Build history of the part. All positions in model axes, mm. Face numbers are marked on the shaded views. A direction names the side the tool comes from. Coordinates: 2 decimals unless noted, no trailing zeros. Loops run counter-clockwise (first coordinate to the right, second up) from the corner with the lowest first, then second, coordinate; pieces in that order, holes last.
Item 1: Flat gauge pins, fed straight in: pin 1 (19 mm diameter, centred on x = 1, y = 11.5, fed in from +Z); pin 2 (10 mm diameter, centred on y = 38.5, z = 6.5, fed in from +X); pin 3 (4 mm diameter, centred on x = -24, z = -1.5, fed in from +Y); pin 4 (10.5 mm diameter, centred on y = 19.5, z = 9.5, fed in from -X). Where does each tip first touch, or does it go through?
Item 2: Cut at A-A (x = 2). List the corners of the cut face in (y, z).
Item 3: 3-axis set-ups, long thin cutter, end or side, ignore diameter. For the marked faces 1, 2, 3, 4 and 5: which of +Z, -Z, +X, -X, +Y, -Y reach the whole face in a straight line?
Item 4: Mould opens along Y. For the marked faces 6, 7 and 8 say: released by +Y, released by -Y, zero draft, split by the parting line, or undercut.
Item 5: Cut at B-B (y = 20). List the corners of the cut face in (x, z).
Item 6: Drill centre lines: line 1 along X through (y, z) = (28, 4.25); line 2 along Z through (x, y) = (27, 4.5); line 3 along X through (y, z) = (5, 0.75). Where is each one in solid material? Low to high.
from build123d import *

# Parameters (mm, degrees)
SKETCH13_W              = 80
SKETCH13_H              = 8
BOSS_EXTRUDE9_DEPTH     = 6.5
SKETCH14_W              = 15
SKETCH14_H              = 3.4999999999999996
CUT_EXTRUDE1_DEPTH      = 41.72161588149469
SKETCH15_W              = 35
SKETCH15_H              = 8
BOSS_EXTRUDE10_DEPTH    = 15
BOSS_EXTRUDE11_DEPTH    = 35
SKETCH17_R              = 3.0000000000000036
SKETCH17_R_2            = 3
BOSS_EXTRUDE12_DEPTH    = 1
SKETCH20_R              = 1.3000000000000023
CUT_EXTRUDE2_DEPTH      = 68.35348577458582
CUT_EXTRUDE3_DEPTH      = 68.33334117794962
CUT_EXTRUDE3_DEPTH_BACK = 68.33334117794962
CUT_EXTRUDE4_DEPTH      = 68.3333411779496
FILLET2_R               = 1.5
CHAMFER1_SIZE           = 1
FILLET3_R               = 20
FILLET4_R               = 2.5


with BuildPart() as part:
    # Sketch13 → Boss-Extrude9 (new body)
    with BuildSketch(Plane(origin=(0, 0, 0), x_dir=(1, 0, 0), z_dir=(0, 1, 0))):
        Rectangle(SKETCH13_W, SKETCH13_H)
    extrude(amount=BOSS_EXTRUDE9_DEPTH)

    # Sketch14 → Cut-Extrude1 (cut, through all)
    with BuildSketch(Plane(origin=(0, 6.5, 0), x_dir=(1, 0, 0), z_dir=(0, 1, 0))):
        Polygon((-35, -1.75), (-20, -1.7499999999999998), (-20, 1.7499999999999998), (-35, 1.75), align=None)
        with Locations((27.5, 0)):
            Rectangle(SKETCH14_W, SKETCH14_H)
    extrude(amount=-CUT_EXTRUDE1_DEPTH, mode=Mode.SUBTRACT)

    # Sketch15 → Boss-Extrude10 (add)
    with BuildSketch(Plane(origin=(0, 6.5, 0), x_dir=(1, 0, 0), z_dir=(0, 1, 0))):
        Rectangle(SKETCH15_W, SKETCH15_H)
    extrude(amount=BOSS_EXTRUDE10_DEPTH)

    # Sketch16 → Boss-Extrude11 (add)
    with BuildSketch(Plane.ZY.offset(17.5)):
        Polygon((4, 21.5), (16.678547852220913, 48.689233611099525), (10.107397413474738, 51.75341138357542), (-4, 21.5), align=None)
    extrude(amount=-BOSS_EXTRUDE11_DEPTH)

    # Sketch17 → Boss-Extrude12 (add)
    with BuildSketch(Plane(origin=(0, 2.307944309631712, -4.949402544155895), x_dir=(1, 0, 0), z_dir=(0, -0.42261826174069717, 0.9063077870366509))):
        with Locations(Location((-10.500000000000005, 47.17609046825079, 0), (0, 0, 90))):
            Circle(SKETCH17_R)
        with Locations(Location((10.499999999999995, 47.17609046825079, 0), (0, 0, 90))):
            Circle(SKETCH17_R_2)
        with Locations(Location((10.499999999999995, 34.67609046825079, 0), (0, 0, 90))):
            Circle(SKETCH17_R_2)
        with Locations(Location((-10.500000000000005, 34.67609046825079, 0), (0, 0, 90))):
            Circle(SKETCH17_R)
    extrude(amount=BOSS_EXTRUDE12_DEPTH)

    # Sketch20 → Cut-Extrude2 (cut, through all)
    with BuildSketch(Plane(origin=(0, 1.885326047891013, -4.043094757119239), x_dir=(1, 0, 0), z_dir=(0, -0.4226182617406972, 0.906307787036651))):
        with Locations(Location((-10.500000000000005, 47.176090468250806, 0), (0, 0, 270))):
            Circle(SKETCH20_R)
        with Locations(Location((10.499999999999995, 47.176090468250806, 0), (0, 0, 270))):
            Circle(SKETCH20_R)
        with Locations(Location((10.499999999999995, 34.67609046825079, 0), (0, 0, 270))):
            Circle(SKETCH20_R)
        with Locations(Location((-10.500000000000005, 34.67609046825079, 0), (0, 0, 270))):
            Circle(SKETCH20_R)
    extrude(amount=-CUT_EXTRUDE2_DEPTH, mode=Mode.SUBTRACT)

    # Sketch21 → Cut-Extrude3 (cut, two sides: drawn at the far end of the back side and taken through both)
    with BuildSketch(Plane(origin=(0, 2.307944309631711, -4.949402544155892), x_dir=(1, 0, 0), z_dir=(0, -0.4226182617406972, 0.906307787036651)).offset(-CUT_EXTRUDE3_DEPTH_BACK)):
        Polygon((-11.500000000000002, 9.676090468250791), (11.499999999999998, 9.676090468250791), (11.499999999999995, 29.67609046825079), (-11.500000000000002, 29.67609046825079), align=None)
    extrude(amount=CUT_EXTRUDE3_DEPTH + CUT_EXTRUDE3_DEPTH_BACK, mode=Mode.SUBTRACT)

    # Sketch22 → Cut-Extrude4 (cut, through all)
    with BuildSketch(Plane(origin=(0, 2.307944309631712, -4.949402544155895), x_dir=(1, 0, 0), z_dir=(0, -0.42261826174069717, 0.9063077870366509))):
        Polygon((-6.000000000000002, 47.676090468250806), (6.000000000000002, 47.676090468250806), (6, 29.676090468250802), (-6, 29.676090468250802), align=None)
    extrude(amount=-CUT_EXTRUDE4_DEPTH, mode=Mode.SUBTRACT)

    # Fillet2
    fillet2_edges = [part.edges().sort_by_distance(p)[0] for p in [
        (-20, 3.25, -1.7499999999999998),
        (-20, 3.25, 1.7499999999999998),
        (-35, 3.25, 1.75),
        (-35, 3.25, -1.75),
        (35, 3.25, -1.7499999999999998),
        (35, 3.25, 1.7499999999999998),
        (20, 3.25, 1.7499999999999998),
        (20, 3.25, -1.7499999999999998),
    ]]
    fillet(fillet2_edges, radius=FILLET2_R)

    # Chamfer1
    chamfer1_edges = [part.edges().sort_by_distance(p)[0] for p in [
        (10.499999999999995, 42.345079101842984, 13.720220020036038),
        (10.499999999999995, 31.016231763884843, 8.437491748277322),
        (-10.500000000000005, 42.345079101842984, 13.720220020036038),
        (-10.500000000000005, 31.01623176388484, 8.43749174827732),
    ]]
    chamfer(chamfer1_edges, length=CHAMFER1_SIZE - 0.0001)  # a hair under: the kernel refuses the full size

    # Fillet3
    fillet3_edges = [part.edges().sort_by_distance(p)[0] for p in [
        (14.5, 21.5, 4),
        (-14.5, 21.5, -4),
        (14.499999999999998, 21.5, -4),
        (-14.5, 21.5, 4),
    ]]
    fillet(fillet3_edges, radius=FILLET3_R)

    # Fillet4
    fillet4_edges = [part.edges().sort_by_distance(p)[0] for p in [
        (11.499999999999998, 10.676384564551352, 0),
        (11.499999999999995, 30.735705076049488, 4.306680005422848),
        (-11.500000000000002, 10.676384564551352, -7.11e-15),
        (-11.500000000000002, 30.735705076049495, 4.306680005422834),
        (-6, 30.7357050760495, 4.306680005422846),
        (6, 30.7357050760495, 4.306680005422846),
        (6.000000000000002, 47.049245242709226, 11.913808716755398),
        (-6.000000000000002, 47.049245242709226, 11.913808716755398),
    ]]
    fillet(fillet4_edges, radius=FILLET4_R)


solid = part.part
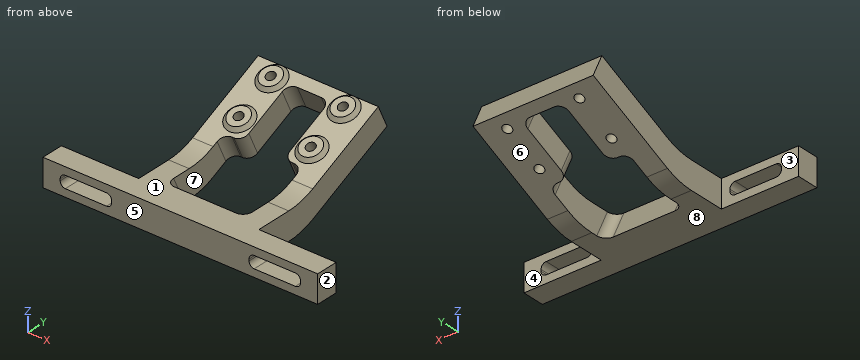
Filled sheet:
1. pin 1: stops at z = 4
1. pin 2: stops at x = 17.5
1. pin 3: stops at y = 6.5
1. pin 4: passes through
2. outline: (0, -4) - (12.54, -4) - (8.81, 4) - (0, 4) - close; (45.52, 15.2) - (48.58, 8.63) - (51.75, 10.11) - (48.69, 16.68) - close
3. face 1: +Z, +X, -X, -Y
3. face 2: +Z, -Z, +X, +Y, -Y
3. face 3: +Z, -Z, -X, +Y
3. face 4: +Z, -Z, +X, +Y
3. face 5: +Z, -Z, +X, -X, -Y
4. face 6: released by +Y
4. face 7: undercut
4. face 8: zero draft
5. outline: (-17.5, -3.78) - (-11.5, -3.78) - (-11.5, 4.22) - (-17.5, 4.22) - close; (11.5, -3.78) - (17.5, -3.78) - (17.5, 4.22) - (11.5, 4.22) - close
6. line 1: x = -17.5 to -11.5, 11.5 to 17.5
6. line 2: z = -4 to -1.75, 1.75 to 4
6. line 3: x = -40 to -34.91, -20.09 to 20.09, 34.91 to 40
